from build123d import *

# Parameters (mm, degrees)
F1_DEPTH = 23.6


with BuildPart() as f1:
    # F0 (on Top) → F1 (new body)
    with BuildSketch(Plane.XY):
        with BuildLine():
            ThreePointArc((-33.1300476876, 66.8774403692), (-29.6868850055, 64.7921543722), (-28.3365694268, 61))
            ThreePointArc((-28.3365694268, 61), (-29.6868850055, 57.2078456278), (-33.1300476876, 55.1225596308))
            ThreePointArc((-33.1300476876, 55.1225596308), (-33.6875488508, 54.042895786), (-34.3365694268, 53.0156402887))
            Line((-34.3365694268, 53.0156402887), (-34.3365694268, 47))
            ThreePointArc((-34.3365694268, 47), (-24.4370744902, 51.1005050634), (-20.3365694268, 61))
            ThreePointArc((-20.3365694268, 61), (-24.4370744902, 70.8994949366), (-34.3365694268, 75))
            ThreePointArc((-34.3365694268, 75), (-37.2771676859, 74.6876908892), (-40.0865694268, 73.7646974112))
            ThreePointArc((-40.0865694268, 73.7646974112), (-35.9867280033, 70.9489006394), (-33.1300476876, 66.8774403692))
        make_face()
        with BuildLine():
            ThreePointArc((-45.8365694268, 75), (-42.8959711677, 74.6876908892), (-40.0865694268, 73.7646974112))
            ThreePointArc((-40.0865694268, 73.7646974112), (-37.2771676859, 74.6876908892), (-34.3365694268, 75))
            Line((-34.3365694268, 75), (-45.8365694268, 75))
        make_face()
        with BuildLine():
            ThreePointArc((-47.0430911659, 66.8774403692), (-44.1864108503, 70.9489006394), (-40.0865694268, 73.7646974112))
            ThreePointArc((-40.0865694268, 73.7646974112), (-42.8959711677, 74.6876908892), (-45.8365694268, 75))
            ThreePointArc((-45.8365694268, 75), (-58.7268044704, 66.4627685766), (-55.8960509898, 51.2631200745))
            ThreePointArc((-55.8960509898, 51.2631200745), (-48.4699754944, 47.2499028191), (-40.0865694268, 48.2353025888))
            ThreePointArc((-40.0865694268, 48.2353025888), (-44.1864108503, 51.0510993606), (-47.0430911659, 55.1225596308))
            ThreePointArc((-47.0430911659, 55.1225596308), (-51.8365694268, 61), (-47.0430911659, 66.8774403692))
        make_face()
        with BuildLine():
            ThreePointArc((-20.3365694268, 61), (-24.4370744902, 51.1005050634), (-34.3365694268, 47))
            Line((-34.3365694268, 47), (-34.3365694268, 0.4321282686))
            add(Edge.make_bspline(
                [(-34.3365694268, 0.4321282686), (-34.3361365089, 0.2880770506), (-34.3361368633, 0.1440338578), (-34.3365694268, 0)],
                knots=[0.496094715, 0.496094715, 0.496094715, 0.496094715, 0.4996371995, 0.4996371995, 0.4996371995, 0.4996371995], degree=3))
            Line((-34.3365694268, 0), (-34.3365694268, -47))
            ThreePointArc((-34.3365694268, -47), (-24.4370744902, -51.1005050634), (-20.3365694268, -61))
            Line((-20.3365694268, -61), (-20.3365694268, 61))
        make_face()
        with BuildLine():
            Line((-34.3365694268, 0.4321282686), (-34.3365694268, 47))
            ThreePointArc((-34.3365694268, 47), (-37.2771676859, 47.3123091108), (-40.0865694268, 48.2353025888))
            ThreePointArc((-40.0865694268, 48.2353025888), (-48.4699754944, 47.2499028191), (-55.8960509898, 51.2631200745))
            add(Edge.make_bspline(
                [(-55.8960509898, 51.2631200745), (-40.9271633104, 35.7982841304), (-34.3895319866, 18.0551513004), (-34.3365694268, 0.4321282686)],
                knots=[0.0627121484, 0.0627121484, 0.0627121484, 0.0627121484, 0.496094715, 0.496094715, 0.496094715, 0.496094715], degree=3))
        make_face()
        with BuildLine():
            add(Edge.make_bspline(
                [(-34.3365694268, 0.4321282686), (-34.3361365089, 0.2880770506), (-34.3361368633, 0.1440338578), (-34.3365694268, 0)],
                knots=[0.496094715, 0.496094715, 0.496094715, 0.496094715, 0.4996371995, 0.4996371995, 0.4996371995, 0.4996371995], degree=3))
            Line((-34.3365694268, 0.4321282686), (-34.3365694268, 0))
        make_face()
        with BuildLine():
            ThreePointArc((-34.3365694268, -75), (-24.4370744902, -70.8994949366), (-20.3365694268, -61))
            ThreePointArc((-20.3365694268, -61), (-24.4370744902, -51.1005050634), (-34.3365694268, -47))
            Line((-34.3365694268, -47), (-34.3365694268, -53.0156402887))
            ThreePointArc((-34.3365694268, -53.0156402887), (-33.6875488508, -54.042895786), (-33.1300476876, -55.1225596308))
            ThreePointArc((-33.1300476876, -55.1225596308), (-29.6868850055, -57.2078456278), (-28.3365694268, -61))
            ThreePointArc((-28.3365694268, -61), (-29.6868850055, -64.7921543722), (-33.1300476876, -66.8774403692))
            ThreePointArc((-33.1300476876, -66.8774403692), (-35.9867280033, -70.9489006394), (-40.0865694268, -73.7646974112))
            ThreePointArc((-40.0865694268, -73.7646974112), (-37.2771676859, -74.6876908892), (-34.3365694268, -75))
        make_face()
        with BuildLine():
            Line((-34.3365694268, -47), (-34.3365694268, 0))
            add(Edge.make_bspline(
                [(-34.3365694268, 0), (-34.3900880153, -17.8204800119), (-41.0597288004, -35.4980627256), (-56.0312077554, -51.4047225497)],
                knots=[0.4996371995, 0.4996371995, 0.4996371995, 0.4996371995, 0.9379284167, 0.9379284167, 0.9379284167, 0.9379284167], degree=3))
            ThreePointArc((-56.0312077554, -51.4047225497), (-48.5660397399, -47.2686493086), (-40.0865694268, -48.2353025888))
            ThreePointArc((-40.0865694268, -48.2353025888), (-37.2771676859, -47.3123091108), (-34.3365694268, -47))
        make_face()
        with BuildLine():
            Line((-45.8365694268, -75), (-34.3365694268, -75))
            ThreePointArc((-34.3365694268, -75), (-37.2771676859, -74.6876908892), (-40.0865694268, -73.7646974112))
            ThreePointArc((-40.0865694268, -73.7646974112), (-42.8959711677, -74.6876908892), (-45.8365694268, -75))
        make_face()
        with BuildLine():
            ThreePointArc((-40.0865694268, -48.2353025888), (-48.5660397399, -47.2686493086), (-56.0312077554, -51.4047225497))
            ThreePointArc((-56.0312077554, -51.4047225497), (-58.6882985771, -66.5527522768), (-45.8365694268, -75))
            ThreePointArc((-45.8365694268, -75), (-42.8959711677, -74.6876908892), (-40.0865694268, -73.7646974112))
            ThreePointArc((-40.0865694268, -73.7646974112), (-44.1864108503, -70.9489006394), (-47.0430911659, -66.8774403692))
            ThreePointArc((-47.0430911659, -66.8774403692), (-51.8365694268, -61), (-47.0430911659, -55.1225596308))
            ThreePointArc((-47.0430911659, -55.1225596308), (-44.1864108503, -51.0510993606), (-40.0865694268, -48.2353025888))
        make_face()
        with BuildLine():
            ThreePointArc((-33.1300476876, -55.1225596308), (-33.6875488508, -54.042895786), (-34.3365694268, -53.0156402887))
            Line((-34.3365694268, -53.0156402887), (-34.3365694268, -55))
            ThreePointArc((-34.3365694268, -55), (-33.730204114, -55.0307185435), (-33.1300476876, -55.1225596308))
        make_face()
        with BuildLine():
            ThreePointArc((-40.0865694268, 62.7139136501), (-37.4178901439, 66.1483456215), (-33.1300476876, 66.8774403692))
            ThreePointArc((-33.1300476876, 66.8774403692), (-35.9867280033, 70.9489006394), (-40.0865694268, 73.7646974112))
            ThreePointArc((-40.0865694268, 73.7646974112), (-44.1864108503, 70.9489006394), (-47.0430911659, 66.8774403692))
            ThreePointArc((-47.0430911659, 66.8774403692), (-42.7552487096, 66.1483456215), (-40.0865694268, 62.7139136501))
        make_face()
        with BuildLine():
            Line((-34.3365694268, 53.0156402887), (-34.3365694268, 55))
            ThreePointArc((-34.3365694268, 55), (-37.922410897, 56.1894136584), (-40.0865694268, 59.2860863499))
            ThreePointArc((-40.0865694268, 59.2860863499), (-42.7552487096, 55.8516543785), (-47.0430911659, 55.1225596308))
            ThreePointArc((-47.0430911659, 55.1225596308), (-44.1864108503, 51.0510993606), (-40.0865694268, 48.2353025888))
            ThreePointArc((-40.0865694268, 48.2353025888), (-36.886511766, 50.2344778172), (-34.3365694268, 53.0156402887))
        make_face()
        with BuildLine():
            Line((-34.3365694268, 47), (-34.3365694268, 53.0156402887))
            ThreePointArc((-34.3365694268, 53.0156402887), (-36.886511766, 50.2344778172), (-40.0865694268, 48.2353025888))
            ThreePointArc((-40.0865694268, 48.2353025888), (-37.2771676859, 47.3123091108), (-34.3365694268, 47))
        make_face()
        with BuildLine():
            ThreePointArc((-47.0430911659, -66.8774403692), (-44.1864108503, -70.9489006394), (-40.0865694268, -73.7646974112))
            ThreePointArc((-40.0865694268, -73.7646974112), (-35.9867280033, -70.9489006394), (-33.1300476876, -66.8774403692))
            ThreePointArc((-33.1300476876, -66.8774403692), (-37.4178901439, -66.1483456215), (-40.0865694268, -62.7139136501))
            ThreePointArc((-40.0865694268, -62.7139136501), (-42.7552487096, -66.1483456215), (-47.0430911659, -66.8774403692))
        make_face()
        with BuildLine():
            Line((-34.3365694268, -53.0156402887), (-34.3365694268, -47))
            ThreePointArc((-34.3365694268, -47), (-37.2771676859, -47.3123091108), (-40.0865694268, -48.2353025888))
            ThreePointArc((-40.0865694268, -48.2353025888), (-36.886511766, -50.2344778172), (-34.3365694268, -53.0156402887))
        make_face()
        with BuildLine():
            Line((-34.3365694268, -55), (-34.3365694268, -53.0156402887))
            ThreePointArc((-34.3365694268, -53.0156402887), (-36.886511766, -50.2344778172), (-40.0865694268, -48.2353025888))
            ThreePointArc((-40.0865694268, -48.2353025888), (-44.1864108503, -51.0510993606), (-47.0430911659, -55.1225596308))
            ThreePointArc((-47.0430911659, -55.1225596308), (-42.7552487096, -55.8516543785), (-40.0865694268, -59.2860863499))
            ThreePointArc((-40.0865694268, -59.2860863499), (-37.922410897, -56.1894136584), (-34.3365694268, -55))
        make_face()
        with BuildLine():
            ThreePointArc((-34.3365694268, 53.0156402887), (-33.6875488508, 54.042895786), (-33.1300476876, 55.1225596308))
            ThreePointArc((-33.1300476876, 55.1225596308), (-33.730204114, 55.0307185435), (-34.3365694268, 55))
            Line((-34.3365694268, 55), (-34.3365694268, 53.0156402887))
        make_face()
    extrude(amount=F1_DEPTH)


solid = f1.part
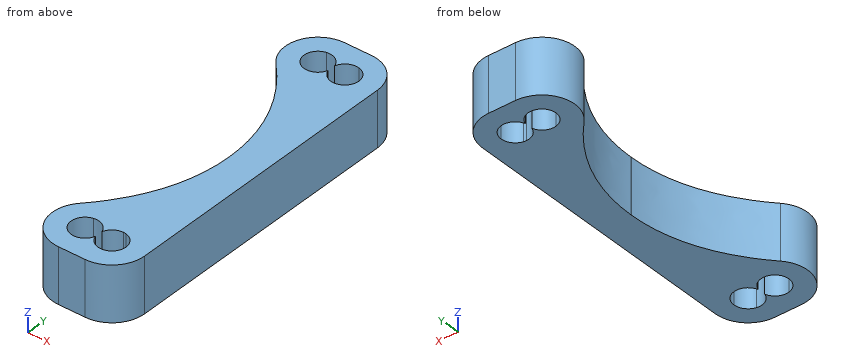
Read the model definition and answer for the solid it produces. Units are mm, in the model's axes. Give positions to 0.01 mm unless a question says otherwise; leave off trailing zeros. Loops run counter-clockwise (first coordinate to the right, second up) from the corner with the lowest first, then second, coordinate; pieces in that order, holes last. Notation, with made-up numbers: (29, -8.5) -> (78, -8.5) arc R9 ccw to (78, 4.5) -> close; hole circle Ø5 at (-8, 11.5). An arc over 180 degrees is marked (long way). Answer as CSV lines item,"result".
Item 1: Each of these flat-tipped pins is pushed along its axis until it touches: pin 1 (1.5 mm diameter, centred on x = -35, y = 53.5, fed in from -Z); pin 2 (4 mm diameter, centred on x = -54.5, z = 14, fed in from +Y); pin 3 (12 mm diameter, centred on x = -55, z = 15.5, fed in from -Y); pin 4 (2 mm diameter, centred on y = 41.5, z = 13.5, fed in from -X). Where does it stop, or does it pass through?
Returned:
pin 1,"stops at z = 0"
pin 2,"stops at y = 73.31"
pin 3,"stops at y = -74.64"
pin 4,"stops at x = -48.47"
Item 2: Find section A-A on x = -37.5. State how many separate pieces and enclosed holes the cut face has, plus the area to 3 significant figures.
Returned:
separate pieces,"4"
enclosed holes,"0"
area,"2,080 mm²"
Item 3: Consider line 1 (X direction, y = -65, z = 19); line 2 (Y direction, x = -46, z = 9); line 3 (Y direction, x = -32.5, z = 15). Determine where each line is inside the solid, lowest interval first. Write a range as [from, to].
Returned:
line 1,"x = [-59.25, -50.31], [-41.36, -38.81], [-29.86, -20.92]"
line 2,"y = [-75, -67], [-55, -38.66], [38.94, 55], [67, 75]"
line 3,"y = [-74.88, -66.71], [-55.29, 55.29], [66.71, 74.88]"
Item 4: Find section D-D on x = -27. Give the vertices of the cut face in (y, z).
Returned:
outline,"(-72.92, 0) -> (72.92, 0) -> (72.92, 23.6) -> (-72.92, 23.6) -> close"
